For this review, take the finished solid that the model builds, in its own axes (mm). Face numbers are marked on the shaded views. A direction names the side the tool comes from. Round coordinates to 2 decimals unless told otherwise and drop trailing zeros. Order: outer loops, then holes, each group sorted by start corner. A loop starts at its lowest first (then second) coordinate and runs counter-clockwise, first axis right, second up. Notation, with made-up numbers: (84.25, -27.75) - (124.25, -27.75) arc R23 cw to (124.25, 3.25) - close; hole circle Ø5 at (49.25, 68). An arc over 180 degrees is marked (long way). One line per question, with ' | ' between items.
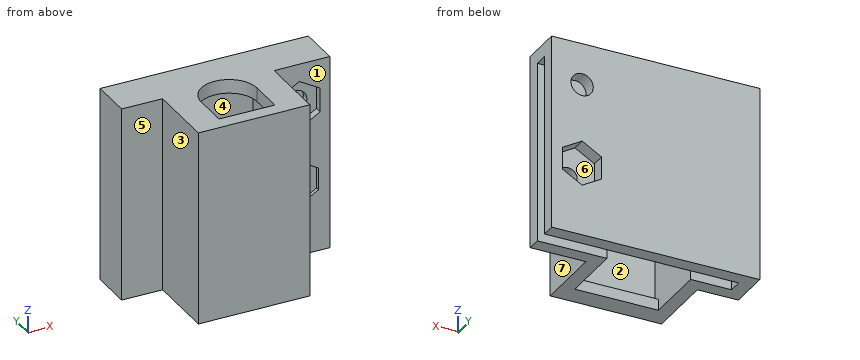
```python
from build123d import *

# Parameters (mm, degrees)
EXTRUDE_1_DEPTH          = 2
EXTRUDE_2_DEPTH          = 26
SKETCH_3_W               = 12
SKETCH_3_H               = 1
EXTRUDE_3_DEPTH          = 1.6
CUT_EXTRUDE_1_DEPTH      = 2
CUT_EXTRUDE_2_DEPTH      = 0.5
CUT_EXTRUDE_3_DEPTH      = 1
CUT_EXTRUDE_4_DEPTH      = 1
CUT_EXTRUDE_4_DEPTH_BACK = 33.449961479
SKETCH_7_R               = 1.35
SKETCH_7_R_2             = 1.6


with BuildPart() as part:
    # 草图1 → 凸台-拉伸1 (new body)
    with BuildSketch(Plane.XY):
        with BuildLine():
            Line((8, -7), (8, 3))
            Line((8, 3), (16, 3))
            Line((16, 3), (16, 5))
            Line((16, 5), (8, 5))
            Line((8, 5), (5, 5))
            ThreePointArc((5, 5), (5.707106781, 4.707106781), (6, 4))
            Line((6, 4), (6, -4))
            ThreePointArc((6, -4), (5.707106781, -4.707106781), (5, -5))
            Line((5, -5), (4, -5))
            Line((4, -5), (-4, -5))
            Line((-4, -5), (-5, -5))
            ThreePointArc((-5, -5), (-5.707106781, -4.707106781), (-6, -4))
            Line((-6, -4), (-6, 4))
            ThreePointArc((-6, 4), (-5.707106781, 4.707106781), (-5, 5))
            Line((-5, 5), (-8, 5))
            Line((-8, 5), (-11.875, 5))
            Line((-11.875, 5), (-11.875, 7))
            Line((-11.875, 7), (16, 7))
            Line((16, 7), (16, 9))
            Line((16, 9), (-13.875, 9))
            Line((-13.875, 9), (-13.875, 3))
            Line((-13.875, 3), (-8, 3))
            Line((-8, 3), (-8, -7))
            Line((-8, -7), (8, -7))
        make_face()
        Polygon((8, 5), (16, 5), (16, 7), (-11.875, 7), (-11.875, 5), (-8, 5), (-5, 5), (5, 5), align=None)
        with BuildLine():
            ThreePointArc((6, 4), (5.707106781, 4.707106781), (5, 5))
            Line((5, 5), (-5, 5))
            ThreePointArc((-5, 5), (-5.707106781, 4.707106781), (-6, 4))
            Line((-6, 4), (-6, -4))
            ThreePointArc((-6, -4), (-5.707106781, -4.707106781), (-5, -5))
            Line((-5, -5), (-4, -5))
            Line((-4, -5), (-4, 0))
            ThreePointArc((-4, 0), (0, 4), (4, 0))
            Line((4, 0), (4, -5))
            Line((4, -5), (5, -5))
            ThreePointArc((5, -5), (5.707106781, -4.707106781), (6, -4))
            Line((6, -4), (6, 4))
        make_face()
    extrude(amount=EXTRUDE_1_DEPTH)

    # 草图2 → 凸台-拉伸2 (add)
    with BuildSketch(Plane(origin=(0, 0, 0), x_dir=(-1, 0, 0), z_dir=(0, 0, -1))):
        Polygon((6, -4), (6, -5), (5, -5), (-5, -5), (-6, -5), (-6, -4), (-6, 4), (-6, 5), (-16, 5), (-16, 3), (-8, 3), (-8, -7), (8, -7), (8, 3), (13.875, 3), (13.875, 9), (-16, 9), (-16, 7), (11.875, 7), (11.875, 5), (6, 5), (6, 4), align=None)
    extrude(amount=EXTRUDE_2_DEPTH)

    # 草图3 → 凸台-拉伸3 (add)
    with BuildSketch(Plane(origin=(0, 0, -26), x_dir=(-1, 0, 0), z_dir=(0, 0, -1))):
        with Locations((0, -4.5)):
            Rectangle(SKETCH_3_W, SKETCH_3_H)
    extrude(amount=-EXTRUDE_3_DEPTH)

    # 草图4 → 切除-拉伸1 (cut)
    with BuildSketch(Plane(origin=(0, 9, 0), x_dir=(1, 0, 0), z_dir=(0, 1, 0))):
        Polygon((11.625, 12.272649731), (14.41996732, 13.886324865), (14.41996732, 17.113675135), (11.625, 18.727350269), (8.83003268, 17.113675135), (8.83003268, 13.886324865), align=None)
    extrude(amount=-CUT_EXTRUDE_1_DEPTH, mode=Mode.SUBTRACT)

    # 草图5 → 切除-拉伸2 (cut)
    with BuildSketch(Plane.XZ.offset(-3)):
        Polygon((11.625, -18.675426481), (14.375, -17.08771324), (14.375, -13.91228676), (11.625, -12.324573519), (8.875, -13.91228676), (8.875, -17.08771324), align=None)
    extrude(amount=-CUT_EXTRUDE_2_DEPTH, mode=Mode.SUBTRACT)

    # 草图6 → 切除-拉伸3 (cut)
    with BuildSketch(Plane.XZ.offset(-3)):
        Polygon((8.625, -5.732050808), (11.625, -7.464101615), (14.625, -5.732050808), (14.625, -2.267949192), (11.625, -0.535898385), (8.625, -2.267949192), align=None)
    extrude(amount=-CUT_EXTRUDE_3_DEPTH, mode=Mode.SUBTRACT)

    # 草图7 → 切除-拉伸4 (cut, two sides: drawn at the far end of the back side and taken through both)
    with BuildSketch(Plane.XZ.offset(-4).offset(-CUT_EXTRUDE_4_DEPTH_BACK)):
        with Locations(Location((11.625, -15.5, 0), (0, 0, 180))):
            Circle(SKETCH_7_R)
        with Locations(Location((11.625, -4, 0), (0, 0, 180))):
            Circle(SKETCH_7_R_2)
    extrude(amount=CUT_EXTRUDE_4_DEPTH + CUT_EXTRUDE_4_DEPTH_BACK, mode=Mode.SUBTRACT)


solid = part.part
```
(1) For probe 1 along Y at (x, z) = (1, -15.5); probe 2 along Y at (x, z) = (-9.75, -2.75); probe 3 along X at (y, z) = (2, -17.5), list the stretches that pass through material, from the lowest coordinate up. Write a range as [from, to].
Output values:
probe 1: [-7, -5], [7, 9] | probe 2: [3, 5], [7, 9] | probe 3: [-8, -6], [6, 8]
(2) We need section D-D on z = -9.75. State the section outline as (x, y) points (3 decimals).
Output values:
outline: (-13.875, 3) - (-8, 3) - (-8, -7) - (8, -7) - (8, 3) - (16, 3) - (16, 5) - (6, 5) - (6, -5) - (-6, -5) - (-6, 5) - (-11.875, 5) - (-11.875, 7) - (16, 7) - (16, 9) - (-13.875, 9) - close
(3) We need section B-B on z = -4. State the section outline as (x, y) points (3 decimals), plus the area to 3 significant figures.
Output values:
outline: (-13.875, 3) - (-8, 3) - (-8, -7) - (8, -7) - (8, 3) - (8.625, 3) - (8.625, 4) - (10.025, 4) - (10.025, 5) - (6, 5) - (6, -5) - (-6, -5) - (-6, 5) - (-11.875, 5) - (-11.875, 7) - (10.025, 7) - (10.025, 9) - (-13.875, 9) - close; (13.225, 4) - (14.625, 4) - (14.625, 3) - (16, 3) - (16, 5) - (13.225, 5) - close; (13.225, 7) - (16, 7) - (16, 9) - (13.225, 9) - close | area: 148 mm^2
(4) Mouldability with a two-part tool opening along Y and no side actions: class the marked faces 5, 6 and 7 as released by +Y, released by -Y, zero draft, split by the parting line, or undercut.
Output values:
face 5: released by -Y | face 6: undercut | face 7: zero draft
(5) Insertion check: pin 1 (1.8 mm diameter, centred on x = 13, z = -3.5, fed in from -Y); pin 2 (0.6 mm diameter, centred on y = -2, z = 1.5, fed in from -X); pin 3 (4.5 mm diameter, centred on x = 11.5, z = -16.5, fed in from -Y). Each pin has a flat end and moves straight along its axis. Give the tip position at first contact, or say it passes through.
Output values:
pin 1: y = 4 | pin 2: x = -8 | pin 3: y = 3
(6) We need section C-C on x = 14. State the section outline as (y, z) points, plus the area to 3 significant figures.
Output values:
outline: (3, -26) - (5, -26) - (5, 0) - (7, 0) - (7, -13.64) - (9, -13.64) - (9, 2) - (3, 2) - (3, -1.91) - (4, -1.91) - (4, -6.09) - (3, -6.09) - (3, -13.7) - (3.5, -13.7) - (3.5, -17.3) - (3, -17.3) - close; (7, -26) - (9, -26) - (9, -17.36) - (7, -17.36) - close | area: 103 mm^2
(7) For the marked faces 1, 2, 3 and 4, list the 3-axis set-ups (+Z, -Z, +X, -X, +Y, -Y) from which the entire face can be reached by the end or side of a thin tool; tool diameter is ignored.
Output values:
face 1: +Z, -Z, +X, -Y | face 2: none | face 3: +Z, -Z, -X, -Y | face 4: -Z, +X
(8) We need section A-A on y = -3.5. State the section outline as (x, z) points.
Output values:
outline: (-8, -26) - (-6, -26) - (-6, 0) - (-4, 0) - (-4, 2) - (-8, 2) - close; (4, 0) - (6, 0) - (6, -26) - (8, -26) - (8, 2) - (4, 2) - close
